```python
from build123d import *

# Parameters (mm, degrees)
F4_R      = 3.25
F6_DEPTH  = 25.4
F5_R      = 13.27112349
F7_DEPTH  = 25.4
F31_DEPTH = 18.5


with BuildPart() as f1:
    # F0 (on Front) → F1 (revolve)
    with BuildSketch(Plane.XZ):
        with BuildLine():
            Line((0, 4.6), (0, -4.6))
            ThreePointArc((0, -4.6), (4.6, 0), (0, 4.6))
        make_face()
    revolve(axis=Axis((0, 0, 0), (0, 0, -1)))

    # F4 (on offset) → F6 (cut)
    with BuildSketch(Plane.XY.offset(3.2766)):
        Circle(F4_R)
    extrude(amount=F6_DEPTH, mode=Mode.SUBTRACT)

    # F5 (on offset) → F7 (cut)
    with BuildSketch(Plane.XY.offset(-4.223)):
        with Locations((-3.4608042333, 0)):
            Circle(F5_R)
    extrude(amount=-F7_DEPTH, mode=Mode.SUBTRACT)

    # F14 (on offset) → F15 (revolve, cut)
    with BuildSketch(Plane.YZ.offset(4.03)):
        with BuildLine():
            Line((0, 1.125), (0, 0))
            Line((0, 0), (0, -1.125))
            ThreePointArc((0, -1.125), (1.125, 0), (0, 1.125))
        make_face()
    revolve(axis=Axis((4.03, 0, 0), (0, 0, 1)), mode=Mode.SUBTRACT)

    # F18 (on offset) → F19 (revolve, cut)
    with BuildSketch(Plane(origin=(-2.015, 3.4900823773, 0), x_dir=(-0.8660254038, -0.5, 0), z_dir=(-0.5, 0.8660254038, 0))):
        with BuildLine():
            Line((0, 1.125), (0, 0))
            Line((0, 0), (0, -1.125))
            ThreePointArc((0, -1.125), (1.125, 0), (0, 1.125))
        make_face()
    revolve(axis=Axis((-2.015, 3.4900823773, 0), (0, 0, 1)), mode=Mode.SUBTRACT)

    # F22 (on offset) → F23 (revolve, cut)
    with BuildSketch(Plane(origin=(-2.015, -3.4900823773, 0), x_dir=(0.8660254038, -0.5, 0), z_dir=(-0.5, -0.8660254038, 0))):
        with BuildLine():
            Line((0, 1.125), (0, 0))
            Line((0, 0), (0, -1.125))
            ThreePointArc((0, -1.125), (1.125, 0), (0, 1.125))
        make_face()
    revolve(axis=Axis((-2.015, -3.4900823773, 0), (0, 0, 1)), mode=Mode.SUBTRACT)

    # F30 (on line) → F31 (cut)
    with BuildSketch(Plane(origin=(1.7017461736, 3.1961051858, -2.4250315045), x_dir=(0.9206065089, -0.3110824678, 0.2360325274), z_dir=(-0.3904915566, -0.7333949731, 0.5564603828))):
        Polygon((1.0608299635, 3.5694248509), (1.8751677126, 4.5393242035), (1.0608299635, 4.8561265068), align=None)
    extrude(amount=F31_DEPTH, mode=Mode.SUBTRACT)


solid = f1.part
```
Input: part model. Units: mm. Frame: model coordinates. Give positions to 0.01 mm unless a question says otherwise; leave off trailing zeros. Order: outer loops, then holes, each group sorted by start corner. A loop starts at its lowest first (then second) coordinate and runs counter-clockwise, first axis right, second up.
1. Cut plane B-B (z = -0.5). Return loops of the section in (x, y) (1 decimal).
Computed:
outline: (-3, -3.4) arc R1 cw (long way) to (-1.5, -4.3) arc R4.6 ccw to (4.5, -0.9) arc R1 cw (long way) to (4.5, 0.9) arc R4.6 ccw to (-1.5, 4.3) arc R1 cw (long way) to (-3, 3.4) arc R4.6 ccw to start
2. Draft query along X for faces 1 (the face through (0, 0, 3.277)), 2 (the face through (1.64, 2.8, 2.67)). Return one class per face: released by +X, released by -X, zero draft, split by the parting line, or undercut.
Computed:
face 1: zero draft
face 2: undercut
3. Pin query (flat end, axial travel): pin 1 Ø4 at (x, y) = (4, 3) entering from -Z; pin 2 Ø1 at (y, z) = (0, -2) entering from +X; pin 3 Ø3 at (y, z) = (-1.5, 2.5) entering from -X. Return the tip coordinate at first contact, or that it passes through.
Computed:
pin 1: stops at z = -3.49
pin 2: stops at x = 4.35
pin 3: stops at x = -4.38
4. Cut plane A-A (x = 1). Return loops of the section in (y, z).
Computed:
outline: (-3.07, 3.28) arc R4.49 ccw to (-1.53, -4.22) - (1.53, -4.22) arc R4.49 ccw to (3.07, 3.28) - (2.04, 3.28) - (1.87, 3.06) - (1.76, 3.28) - close
5. Cut plane D-D (x = 3.5). Return loops of the section in (y, z).
Computed:
outline: circle Ø5.97 at (0, 0); hole circle Ø1.98 at (0, 0)
6. Cut plane C-C (y = -0.25). Return loops of the section in (x, z).
Computed:
outline: (-3.22, 3.28) arc R4.59 ccw to (-1.81, -4.22) - (1.81, -4.22) arc R4.59 ccw to (4.48, -1) arc R1.1 cw (long way) to (4.48, 1) arc R4.59 ccw to (3.22, 3.28) - close
7. Line query: probe 1 along X at (y, z) = (-3.25, 0.5); probe 2 along Z at (x, y) = (3.5, 0); probe 3 along Z at (x, y) = (-2.5, 2.75). Output: solid intervals per line, ascending.
Computed:
probe 1: x = -3.22 to -2.99, -1.04 to 3.22
probe 2: z = -2.98 to -0.99, 0.99 to 2.98
probe 3: z = -2.71 to -0.69, 0.69 to 2.71
